The listing builds one solid part. Answer for the finished solid, in the listing's coordinates (mm). A direction names the side the tool comes from. Give positions to 0.01 mm unless a question says otherwise; leave off trailing zeros. Loops run counter-clockwise (first coordinate to the right, second up) from the corner with the lowest first, then second, coordinate; pieces in that order, holes last. Notation, with made-up numbers: (72, -33.5) - (103, -33.5) arc R18 cw to (103, -15.5) - close; hole circle Ø9 at (17.25, 64). An arc over 180 degrees is marked (long way). Write each question's results on one line, items separated by ' | '.
from build123d import *

# Parameters (mm, degrees)
SKETCH2_W           = 80
SKETCH2_H           = 117
BOSS_EXTRUDE1_DEPTH = 70
SKETCH3_W           = 80
SKETCH3_H           = 71
CUT_EXTRUDE1_DEPTH  = 65
SKETCH4_W           = 20
SKETCH4_H           = 55
CUT_EXTRUDE2_DEPTH  = 65
CUT_EXTRUDE3_DEPTH  = 143.088000901
SKETCH6_R           = 3
CUT_EXTRUDE4_DEPTH  = 65
SKETCH8_W           = 10
SKETCH8_H           = 117
CUT_EXTRUDE5_DEPTH  = 98.731980436


with BuildPart() as part:
    # Sketch2 → Boss-Extrude1 (new body)
    with BuildSketch(Plane(origin=(0, 0, 0), x_dir=(1, 0, 0), z_dir=(0, 1, 0))):
        Rectangle(SKETCH2_W, SKETCH2_H)
    extrude(amount=BOSS_EXTRUDE1_DEPTH)

    # Sketch3 → Cut-Extrude1 (cut)
    with BuildSketch(Plane(origin=(0, 70, 0), x_dir=(1, 0, 0), z_dir=(0, 1, 0))):
        with Locations((0, 13)):
            Rectangle(SKETCH3_W, SKETCH3_H)
    extrude(amount=-CUT_EXTRUDE1_DEPTH, mode=Mode.SUBTRACT)

    # Sketch4 → Cut-Extrude2 (cut)
    with BuildSketch(Plane.XY.offset(58.5)):
        with Locations((0, 32.5)):
            Rectangle(SKETCH4_W, SKETCH4_H)
    extrude(amount=-CUT_EXTRUDE2_DEPTH, mode=Mode.SUBTRACT)

    # Sketch5 → Cut-Extrude3 (cut, through all)
    with BuildSketch(Plane.XY.offset(58.5)):
        with BuildLine():
            Line((-6.157789331, 65.187529324), (-40, 38.738971621))
            Line((-40, 38.738971621), (-40, 70))
            Line((-40, 70), (40, 70))
            Line((40, 70), (40, 38.738971621))
            Line((40, 38.738971621), (6.157789331, 65.187529324))
            ThreePointArc((6.157789331, 65.187529324), (0, 67.30833961), (-6.157789331, 65.187529324))
        make_face()
    extrude(amount=-CUT_EXTRUDE3_DEPTH, mode=Mode.SUBTRACT)

    # Sketch6 → Cut-Extrude4 (cut)
    with BuildSketch(Plane.XY.offset(-48.5)):
        with Locations((0, 42.2)):
            Circle(SKETCH6_R)
    extrude(amount=-CUT_EXTRUDE4_DEPTH, mode=Mode.SUBTRACT)

    # Sketch8 → Cut-Extrude5 (cut, through all)
    with BuildSketch(Plane(origin=(0, 67.3, 0), x_dir=(1, 0, 0), z_dir=(0, 1, 0))):
        with Locations((-35, 0)):
            Rectangle(SKETCH8_W, SKETCH8_H)
        with Locations((35, 0)):
            Rectangle(SKETCH8_W, SKETCH8_H)
    extrude(amount=-CUT_EXTRUDE5_DEPTH, mode=Mode.SUBTRACT)


solid = part.part
Item 1: A cutting plane is placed at B-B, the plane x = 0. Determine the outline of the cut face in (y, z).
Values found:
outline: (0, -58.5) - (39.2, -58.5) - (39.2, -48.5) - (5, -48.5) - (5, 58.5) - (0, 58.5) - close; (45.2, -58.5) - (67.31, -58.5) - (67.31, -48.5) - (45.2, -48.5) - close; (60, 22.5) - (67.31, 22.5) - (67.31, 58.5) - (60, 58.5) - close
Item 2: A flat-ended cylindrical pin translates along its axis: P1, Ø8, axis at x = -24, z = 15, coming from the +Y side. Find the tip coordinate at first contact, or state that the pin passes through.
Values found:
P1: stops at y = 5
Item 3: Find the intervals of material crossed by line 1 along Z through (x, y) = (-18, 42.5); line 2 along X through (y, z) = (25, 44.5); line 3 along Y through (x, z) = (0, -56), in increasing order. Write a range as [from, to].
Values found:
line 1: z = [-58.5, -48.5], [22.5, 58.5] | line 2: x = [-30, -10], [10, 30] | line 3: y = [0, 39.2], [45.2, 67.31]
Item 4: For a pull along Y with two mould halves and no side action, classify faces 6 (the face through (-10, 32, 41)), 7 (the face through (18.246, 55.74, 40.752)), 8 (the face through (0, 0, -1)) as released by +Y, released by -Y, zero draft, split by the parting line, or undercut.
Values found:
face 6: undercut | face 7: released by +Y | face 8: released by -Y
Item 5: A cutting plane is placed at C-C, the plane z = 26.5. Determine the outline of the cut face in (x, y), plus the area to 3 significant figures.
Values found:
outline: (-30, 0) - (30, 0) - (30, 46.55) - (6.16, 65.19) arc R10 ccw to (-6.16, 65.19) - (-30, 46.55) - close; hole (-10, 5) - (10, 5) - (10, 60) - (-10, 60) - close | area: 2,380 mm²
Item 6: A cutting plane is placed at A-A, the plane y = 42.2. Determine the outline of the cut face in (x, z), plus the area to 3 significant figures.
Values found:
outline: (-30, -58.5) - (-3, -58.5) - (-3, -48.5) - (-30, -48.5) - close; (-30, 22.5) - (-10, 22.5) - (-10, 58.5) - (-30, 58.5) - close; (3, -58.5) - (30, -58.5) - (30, -48.5) - (3, -48.5) - close; (10, 22.5) - (30, 22.5) - (30, 58.5) - (10, 58.5) - close | area: 1,980 mm²
Item 7: For faces 1 (the face through (10, 32, 41)), 2 (the face through (-14, 30, 22.5)), 3 (the face through (0, 5, -8)), 4 (the face through (-17.912, 56.001, -53.43)), 5 (the face through (-0.391, 45.174, -53.43)), determine the directions among +Z, -Z, +X, -X, +Y, -Y from which every point of the face is accessible in a straight line to the end or side of a thin tool.
Values found:
face 1: +Z | face 2: +X, -X, +Y | face 3: none | face 4: +Z, -Z, -X, +Y | face 5: +Z, -Z
Item 8: A cutting plane is placed at D-D, the plane y = 25. Determine the outline of the cut face in (x, z).
Values found:
outline: (-30, -58.5) - (30, -58.5) - (30, -48.5) - (-30, -48.5) - close; (-30, 22.5) - (-10, 22.5) - (-10, 58.5) - (-30, 58.5) - close; (10, 22.5) - (30, 22.5) - (30, 58.5) - (10, 58.5) - close
